```python
from build123d import *

# Parameters (mm, degrees)
F0_W       = 88.9
F0_H       = 88.9
F1_DEPTH   = 88.9
F2_R       = 9.525
F3_DEPTH   = 2.54
F4_R       = 9.525
F5_DEPTH   = 2.54
F6_R       = 9.525
F7_DEPTH   = 2.54
F8_R       = 9.525
F1_FACE1_W = 88.9
F1_FACE1_H = 88.9
F1_FACE1_R = 9.525
F9_DEPTH   = 2.54
F10_R      = 9.525
F11_DEPTH  = 2.54
F12_R      = 9.525
F13_DEPTH  = 2.54
F14_R      = 5.08


with BuildPart() as f1:
    # F0 (on Top) → F1 (new body)
    with BuildSketch(Plane.XY):
        with Locations((44.45, -44.45)):
            Rectangle(F0_W, F0_H)
    extrude(amount=F1_DEPTH)

    # F2 (on face) → F3 (cut)
    with BuildSketch(Plane.XY.offset(88.9)):
        with Locations((22.225, -22.225)):
            Circle(F2_R)
        with Locations((66.675, -22.225)):
            Circle(F2_R)
        with Locations((66.675, -44.45)):
            Circle(F2_R)
        with Locations((22.225, -44.45)):
            Circle(F2_R)
        with Locations((22.225, -66.675)):
            Circle(F2_R)
        with Locations((66.675, -66.675)):
            Circle(F2_R)
    extrude(amount=-F3_DEPTH, mode=Mode.SUBTRACT)

    # F4 (on face) → F5 (cut)
    with BuildSketch(Plane.XZ.offset(88.9)):
        with Locations((22.225, 66.675)):
            Circle(F4_R)
        with Locations((66.675, 66.675)):
            Circle(F4_R)
        with Locations((66.675, 22.225)):
            Circle(F4_R)
        with Locations((22.225, 22.225)):
            Circle(F4_R)
    extrude(amount=-F5_DEPTH, mode=Mode.SUBTRACT)

    # F6 (on face) → F7 (cut)
    with BuildSketch(Plane(origin=(0, 0, 0), x_dir=(1, 0, 0), z_dir=(0, 0, -1))):
        with Locations((44.45, 44.45)):
            Circle(F6_R)
    extrude(amount=-F7_DEPTH, mode=Mode.SUBTRACT)

    # F8 (on face) + F1_face1 (on face) → F9 (cut)
    with BuildSketch(Plane(origin=(0, 0, 0), x_dir=(-1, 0, 0), z_dir=(0, 1, 0))):
        with Locations((-66.675, 66.675)):
            Circle(F8_R)
        with Locations((-44.45, 44.45)):
            Circle(F8_R)
        with Locations((-22.225, 22.225)):
            Circle(F8_R)
    with BuildSketch(Plane(origin=(44.45, -88.9, 44.45), x_dir=(1, 0, 0), z_dir=(0, -1, 0))):
        Rectangle(F1_FACE1_W, F1_FACE1_H)
        with Locations((-22.225, 22.225)):
            Circle(F1_FACE1_R, mode=Mode.SUBTRACT)
        with Locations((22.225, 22.225)):
            Circle(F1_FACE1_R, mode=Mode.SUBTRACT)
        with Locations((-22.225, -22.225)):
            Circle(F1_FACE1_R, mode=Mode.SUBTRACT)
        with Locations((22.225, -22.225)):
            Circle(F1_FACE1_R, mode=Mode.SUBTRACT)
    extrude(amount=-F9_DEPTH, dir=(0, 1, 0), mode=Mode.SUBTRACT)

    # F10 (on face) → F11 (cut)
    with BuildSketch(Plane.YZ.offset(88.9)):
        with Locations((-66.675, 66.675)):
            Circle(F10_R)
        with Locations((-22.225, 66.675)):
            Circle(F10_R)
        with Locations((-44.45, 44.45)):
            Circle(F10_R)
        with Locations((-66.675, 22.225)):
            Circle(F10_R)
        with Locations((-22.225, 22.225)):
            Circle(F10_R)
    extrude(amount=-F11_DEPTH, mode=Mode.SUBTRACT)

    # F12 (on face) → F13 (cut)
    with BuildSketch(Plane(origin=(0, 0, 0), x_dir=(0, -1, 0), z_dir=(-1, 0, 0))):
        with Locations((22.225, 66.675)):
            Circle(F12_R)
        with Locations((66.675, 22.225)):
            Circle(F12_R)
    extrude(amount=-F13_DEPTH, mode=Mode.SUBTRACT)

    # F14
    f14_edges = [f1.edges().sort_by_distance(p)[0] for p in [
        (0, -44.45, 88.9),
        (44.45, -88.9, 88.9),
        (0, -88.9, 44.45),
        (44.45, -88.9, 0),
        (0, -44.45, 0),
        (44.45, 0, 0),
        (0, 0, 44.45),
        (44.45, 0, 88.9),
        (88.9, 0, 44.45),
        (88.9, -44.45, 88.9),
        (88.9, -88.9, 44.45),
        (88.9, -44.45, 0),
    ]]
    fillet(f14_edges, radius=F14_R)


solid = f1.part
```
Geometry: final body of the model. Coordinates: model frame, mm. A direction names the side the tool comes from. Give positions to 0.01 mm unless a question says otherwise; leave off trailing zeros. Order: outer loops, then holes, each group sorted by start corner. A loop starts at its lowest first (then second) coordinate and runs counter-clockwise, first axis right, second up. Notation, with made-up numbers: M 61.5,69 L 65.5,69 A32 ccw 65.5,106 Z; hole C 53.25,36 d7. An arc over 180 degrees is marked long. Answer as CSV lines item,"result". Start each with the question number.
1) Cut plane B-B (z = 44.45). Output: boundary loops of the cut face in (x, y) (3 decimals).
2) Line query: line 1 (X direction, y = -44, z = 87); line 2 (Z direction, x = 57.5, y = -67.5); line 3 (Y direction, x = 60, z = 19.5). Output: solid intervals per line, ascending. Write a range as from..to.
3) Cut plane C-C (x = 44.45). Output: boundary loops of the cut face in (y, z) (3 decimals).
4) Set-up query: faces 4 (the flat face through (67, -2.54, 67)), 5 (the flat face through (86.36, -22, 67)), 6 (the flat face through (67, -22, 86.36)), 7 (the cylindrical face through (37.43, -50.89, 1.25)), 8 (the flat face through (22, -86.36, 67)). Return all of +Z, -Z, +X, -X, +Y, -Y with unobstructed straight access to the full face (end or side cutting, diameter ignored); none if empty.
5) Mould query, pull axis X, two halves, no side actions, for faces 1 (the flat face through (86.36, -67, 22)), 2 (the flat face through (44, -45, 2.54)), 3 (the cylindrical face through (45.001, -87.451, 87.372)). Classes: +X half, -X half, draft (parallel to the pull), parting line (faces both ways), or undercut.
6) Cut plane A-A (y = -44.45). Output: boundary loops of the cut face in (x, z) (3 decimals), then the cut area to 3 significant figures.
7) First-contact query: P1, Ø22, axis at x = 22.225, y = -66.675, coming from the +Z side; P2, Ø1.5, axis at x = 15.5, y = -47.5, coming from the +Z side; P3, Ø5.5, axis at y = -23, z = 70, coming from the -X side; P4, Ø5.5, axis at x = 27, z = 70.5, coming from the -Y side. Flat tips, straight axial feed; report the tip coordinate or a pass-through.
Findings below:
1,outline,"M 0,-83.82 A5.08 ccw 5.08,-88.9 L 83.82,-88.9 A5.08 ccw 88.9,-83.82 L 88.9,-53.975 L 86.36,-53.975 L 86.36,-34.925 L 88.9,-34.925 L 88.9,-5.08 A5.08 ccw 83.82,0 L 53.975,0 L 53.975,-2.54 L 34.925,-2.54 L 34.925,0 L 5.08,0 A5.08 ccw 0,-5.08 Z"
2,line 1,"x = 1.12..12.71, 31.74..57.16, 76.19..87.78"
2,line 2,"z = 0..86.36"
2,line 3,"y = -86.36..0"
3,outline,"M -88.9,5.08 A5.08 ccw -83.82,0 L -53.975,0 L -53.975,2.54 L -34.925,2.54 L -34.925,0 L -5.08,0 A5.08 ccw 0,5.08 L 0,34.925 L -2.54,34.925 L -2.54,53.975 L 0,53.975 L 0,83.82 A5.08 ccw -5.08,88.9 L -83.82,88.9 A5.08 ccw -88.9,83.82 Z"
4,face 4,"+Y"
4,face 5,"+X"
4,face 6,"+Z"
4,face 7,"-Z"
4,face 8,"-Y"
5,face 1,"+X half"
5,face 2,"undercut"
5,face 3,"draft"
6,outline,"M 0,5.08 A5.08 ccw 5.08,0 L 34.925,0 L 34.925,2.54 L 53.975,2.54 L 53.975,0 L 83.82,0 A5.08 ccw 88.9,5.08 L 88.9,34.925 L 86.36,34.925 L 86.36,53.975 L 88.9,53.975 L 88.9,83.82 A5.08 ccw 83.82,88.9 L 76.2,88.9 L 76.2,86.36 L 57.15,86.36 L 57.15,88.9 L 31.75,88.9 L 31.75,86.36 L 12.7,86.36 L 12.7,88.9 L 5.08,88.9 A5.08 ccw 0,83.82 Z"
6,area,"7,690 mm²"
7,P1,"stops at z = 88.9"
7,P2,"stops at z = 86.36"
7,P3,"stops at x = 2.54"
7,P4,"stops at y = -86.36"
